Design review of the part shown in the three views and the two pictorial views. Dimensions are in mm from the part's minimum x, y and z. A direction names the side the tool comes from. Coordinates: 2 decimals unless noted, no trailing zeros. Write each loop counter-clockwise with the first axis right and the second up, starting at its lowest first coordinate (ties: lowest second). Pieces come first, ordered by that corner, then holes.
Q1. For pin 1 Ø4 at (x, y) = (27.5, 5) entering from -Z; pin 2 Ø1 at (x, y) = (6.5, 4) entering from +Z; pin 3 Ø4 at (x, y) = (22, 15) entering from +Z, all flat-tipped, find the tip position at first contact; note any pin that passes through.
Q2. For the marked faces 1, 2, 3 and 4, list the 3-axis set-ups (+Z, -Z, +X, -X, +Y, -Y) from which the entire face can be reached by the end or side of a thin tool; tool diameter is ignored.
Q3. Take a section at A-A, the plane y = 5. State how many separate pieces and enclosed holes the cut face has, plus the area to 3 significant figures.
Q4. Take a section at C-C, the plane x = 3.5. Write out the cut boundary in (y, z), plus the area to 3 significant figures.
Q5. The part is to be moulded in two halves that separate along X. For the marked faces 5, 6 and 7, say which applies: released by +X, released by -X, zero draft, split by the parting line, or undercut.
Q6. Take a section at D-D, the plane x = 24.5. Write out the cut boundary in (y, z).
Q7. For L1, parallel to Z at x = 25.4, y = 11 (1 decimal); L2, parallel to Z at x = 26.5, y = 3.5 (1 decimal); L3, parallel to X at y = 5.5, z = 13 (1 decimal), list the stretches that pass through material, from the lowest coordinate up.
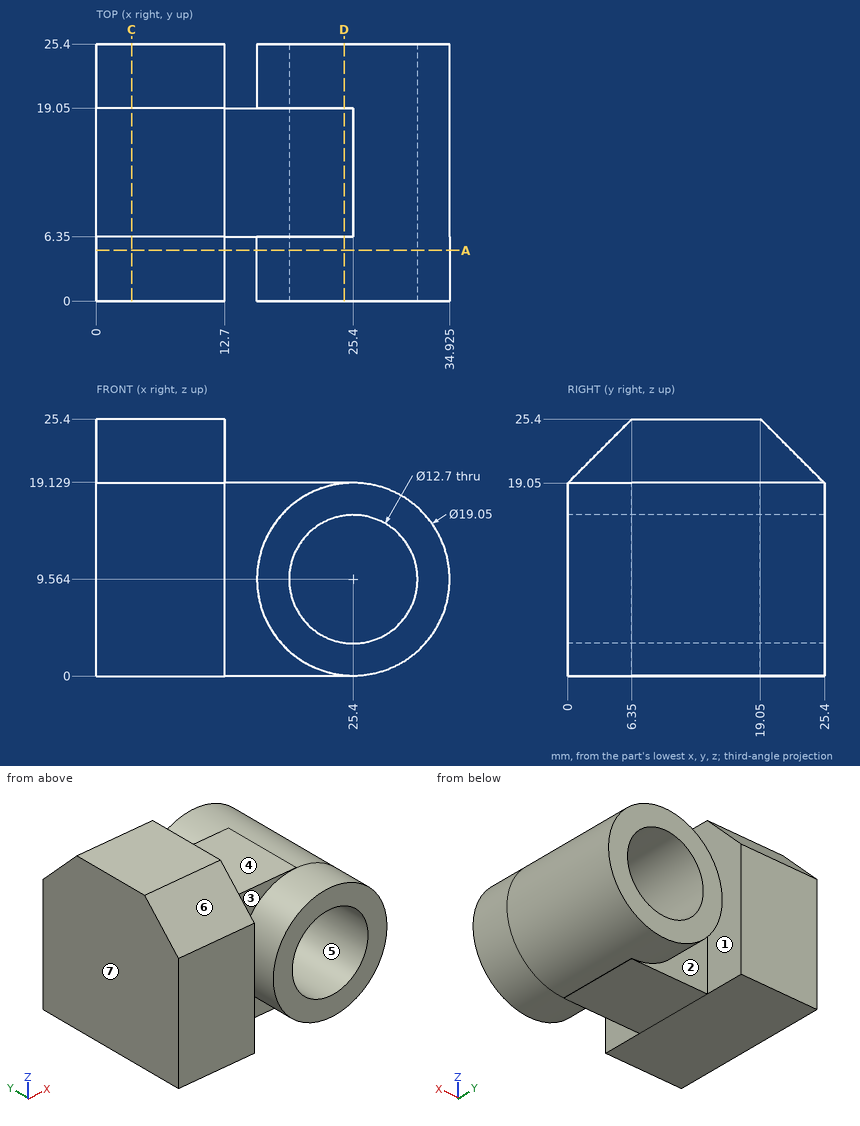
Responses:
1. pin 1: stops at z = 0.04
1. pin 2: stops at z = 23.55
1. pin 3: stops at z = 19.13
2. face 1: +Z
2. face 2: +Y
2. face 3: -Y
2. face 4: +Z, +X, +Y, -Y
3. separate pieces: 2
3. enclosed holes: 1
3. area: 464 mm2
4. outline: (0, 0) - (25.4, 0) - (25.4, 19.05) - (19.05, 25.4) - (6.35, 25.4) - (0, 19.05) - close
4. area: 605 mm2
5. face 5: undercut
5. face 6: zero draft
5. face 7: released by -X
6. outline: (0, 0.08) - (6.35, 0.08) - (6.35, 0) - (19.05, 0) - (19.05, 0.08) - (25.4, 0.08) - (25.4, 3.28) - (0, 3.28) - close; (0, 15.85) - (25.4, 15.85) - (25.4, 19.05) - (19.05, 19.05) - (19.05, 19.13) - (6.35, 19.13) - (6.35, 19.05) - (0, 19.05) - close
7. L1: z = 0 to 3.2, 15.9 to 19.1
7. L2: z = 0.1 to 3.3, 15.8 to 19
7. L3: x = 0 to 12.7, 16.5 to 20.1, 30.7 to 34.3
